```python
from build123d import *

# Parameters (mm, degrees)
SKETCH1_R           = 1
BOSS_EXTRUDE1_DEPTH = 3
SKETCH2_R           = 3
SKETCH2_R_2         = 1
SKETCH2_R_3         = 4
BOSS_EXTRUDE2_DEPTH = 0.5


with BuildPart() as part:
    # Sketch1 → Boss-Extrude1 (new body)
    with BuildSketch(Plane.XY):
        with BuildLine():
            ThreePointArc((-2.645751311, -3), (-1.372549714, -3.757140839), (0.088888889, -3.999012224))
            Line((0.088888889, -3.999012224), (45.066666667, -2.999259168))
            ThreePointArc((45.066666667, -2.999259168), (48, 0), (45.066666667, 2.999259168))
            Line((45.066666667, 2.999259168), (0.088888889, 3.999012224))
            ThreePointArc((0.088888889, 3.999012224), (-1.372549714, 3.757140839), (-2.645751311, 3))
            Line((-2.645751311, 3), (-10, 3))
            ThreePointArc((-10, 3), (-13, 0), (-10, -3))
            Line((-10, -3), (-2.645751311, -3))
        make_face()
        Circle(SKETCH1_R, mode=Mode.SUBTRACT)
        with Locations((-10, 0)):
            Circle(SKETCH1_R, mode=Mode.SUBTRACT)
        with Locations((45, 0)):
            Circle(SKETCH1_R, mode=Mode.SUBTRACT)
    extrude(amount=BOSS_EXTRUDE1_DEPTH)

    # Sketch2 → Boss-Extrude2 (add)
    with BuildSketch(Plane(origin=(0, 0, 0), x_dir=(-1, 0, 0), z_dir=(0, 0, -1))):
        with Locations((10, 0)):
            Circle(SKETCH2_R)
        with Locations((10, 0)):
            Circle(SKETCH2_R_2, mode=Mode.SUBTRACT)
        Circle(SKETCH2_R_3)
        Circle(SKETCH2_R_2, mode=Mode.SUBTRACT)
    extrude(amount=BOSS_EXTRUDE2_DEPTH)


solid = part.part
```
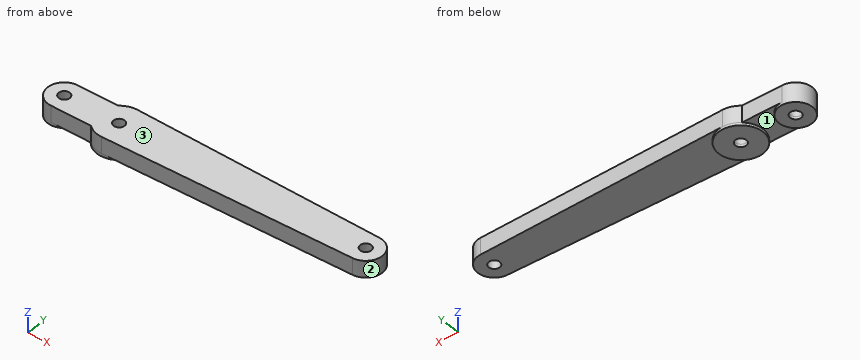
Model file for the job. Use its own axes, mm. Face numbers are marked on the shaded views. Coordinates: 2 decimals unless noted, no trailing zeros. Loops run counter-clockwise (first coordinate to the right, second up) from the corner with the lowest first, then second, coordinate; pieces in that order, holes last. Notation, with made-up numbers: M 76,49 L 91,49 A5 cw 91,55 Z; hole C 54.25,-32 d5. An arc over 180 degrees is marked long. Use CSV: the item, a comma, the result in double quotes. Start each with the question number.
1. Band-saw the part on D-D, the plane x = -8. List the corners of the cut face in (y, z), then the cut area to 3 significant figures.
2. Probe probe 1 along Y at (x, z) = (-10, -0.1); probe 2 along Y at (x, z) = (0, 1.05); probe 3 along X at (y, z) = (0, -0.05). List the from-to ranges inside material, lowest first. Write a range as [from, to].
3. Band-saw the part on B-B, the plane y = 1.75. List the corners of the cut face in (x, z), then the cut area to 3 significant figures.
4. Flat gauge pins, fed straight in: pin 1 (1.5 mm diameter, centred on x = 23.5, z = 1.5, fed in from -Y); pin 2 (1.2 mm diameter, centred on x = 45, y = 0, fed in from +Z); pin 3 (1.8 mm diameter, centred on x = -5.5, y = -1, fed in from -Z); pin 4 (1.5 mm diameter, centred on y = -2, z = 0, fed in from +X). Where does each tip first touch, or does it go through?
5. Band-saw the part on A-A, the plane z = 0.5. List the corners of the cut face in (x, y), then the cut area to 3 significant figures.
6. Two-plate mould, pull along X, no slides. Class the marked faces 1, 2 and 3: pulls with the +X half, pulls with the -X half, needs draft (parallel to the pull), parting line crosses it, or undercut.
7. Band-saw the part on C-C, the plane x = 3.5. List the corners of the cut face in (y, z), then the cut area to 3 significant figures.
Entries:
1,outline,"M -3,0 L -2.24,0 L -2.24,-0.5 L 2.24,-0.5 L 2.24,0 L 3,0 L 3,3 L -3,3 Z"
1,area,"20.2 mm2"
2,probe 1,"y = [-3, -1], [1, 3]"
2,probe 2,"y = [-4, -1], [1, 4]"
2,probe 3,"x = [-13, -11], [-9, -7], [-4, -1], [1, 4]"
3,outline,"M -12.44,-0.5 L -7.56,-0.5 L -7.56,0 L -3.6,0 L -3.6,-0.5 L 3.6,-0.5 L 3.6,0 L 47.44,0 L 47.44,3 L -12.44,3 Z"
3,area,"186 mm2"
4,pin 1,"stops at y = -3.5"
4,pin 2,"passes through"
4,pin 3,"stops at z = 0"
4,pin 4,"stops at x = 47.73"
5,outline,"M -10,-3 L -2.65,-3 A4 ccw 0.09,-4 L 45.07,-3 A3 ccw 45.07,3 L 0.09,4 A4 ccw -2.65,3 L -10,3 A3 ccw Z; hole C -10,0 d2; hole C 0,0 d2; hole C 45,0 d2"
5,area,"398 mm2"
6,face 1,"undercut"
6,face 2,"pulls with the +X half"
6,face 3,"needs draft"
7,outline,"M -3.92,0 L -1.94,0 L -1.94,-0.5 L 1.94,-0.5 L 1.94,0 L 3.92,0 L 3.92,3 L -3.92,3 Z"
7,area,"25.5 mm2"
